Geometry check sheet. Reference: the model listing, model coordinates, mm. Coordinates: 2 decimals unless noted, no trailing zeros. Write each loop counter-clockwise with the first axis right and the second up, starting at its lowest first coordinate (ties: lowest second). Pieces come first, ordered by that corner, then holes. Notation, with made-up numbers: M 88.5,48.5 L 139.5,48.5 A23 ccw 139.5,56.5 Z; hole C 77.5,71.5 d8. An arc over 180 degrees is marked long. Answer as a JSON object with one key per item and string values. Group by question number.
Autodesk Inventor part; units mm, degrees
ref_plane "YZ Plane" through (0, 0, 0) normal (1, 0, 0) x (0, 1, 0)
ref_plane "XZ Plane" through (0, 0, 0) normal (0, 1, 0) x (-1, 0, 0)
ref_plane "XY Plane" through (0, 0, 0) normal (0, 0, 1) x (1, 0, 0)
sketch "Sketch1" plane through (0, 0, 0) normal (0, 0, 1) x (1, 0, 0)
  line L0 (0, 0) -> (101.6, 0)
  line L1 (101.6, 0) -> (101.6, 50.8)
  line L2 (0, 50.8) -> (0, 0)
  line L3 (50.8, 152.4) -> (0, 152.4)
  line L4 (0, 152.4) -> (0, 50.8)
  line L5 (50.8, 152.4) -> (101.6, 50.8)
  circle A0 centre (12.7, 12.7) radius 3.2512
  circle A1 centre (12.7, 38.1) radius 3.2512
  circle A2 centre (12.7, 63.5) radius 3.2512
  circle A3 centre (12.7, 88.9) radius 3.2512
  circle A4 centre (12.7, 114.3) radius 3.2512
  circle A5 centre (12.7, 139.7) radius 3.2512
  circle A6 centre (38.1, 12.7) radius 3.2512
  circle A7 centre (38.1, 38.1) radius 3.2512
  circle A8 centre (38.1, 63.5) radius 3.2512
  circle A9 centre (38.1, 88.9) radius 3.2512
  circle A10 centre (38.1, 114.3) radius 3.2512
  circle A11 centre (38.1, 139.7) radius 3.2512
  circle A12 centre (63.5, 12.7) radius 3.2512
  circle A13 centre (88.9, 12.7) radius 3.2512
  circle A14 centre (38.1, 38.1) radius 3.2512
  circle A15 centre (63.5, 38.1) radius 3.2512
  circle A16 centre (88.9, 38.1) radius 3.2512
  dimension "d6" = 101.6
  dimension "d7" = 50.8
  dimension "d8" = 50.8
  dimension "d9" = 101.6
  dimension "d10" = 50.8
  dimension "d11" = 101.6
  dimension "d12" = 50.8
  dimension "d13" = 6.5024
  dimension "d14" = 12.7
  dimension "d15" = 12.7
  dimension "d18" = 25.4
  dimension "d21" = 25.4
  dimension "d26" = 25.4
  dimension "d29" = 25.4
extrude "Extrusion1" add sketch "Sketch1" along normal blind 6.35
properties part number "6x4"
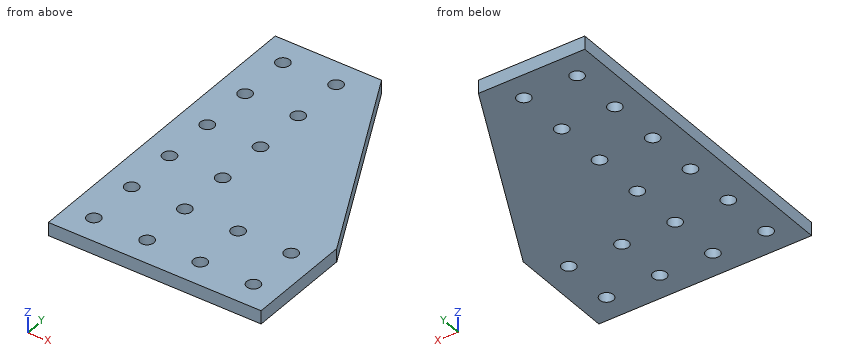
1) Material ranges on probe 1 along Y at (x, z) = (62, 4); probe 2 along Y at (x, z) = (78, 2.25); probe 3 along Y at (x, z) = (77, 1.75), recorded low to high. Write a range as [from, to].
2) Section check A-A (y = 12.7). Record the cut outline in (x, z), then the cut area to 3 significant figures.
3) Section check B-B (x = 63.5). Record the cut outline in (y, z), then the cut area to 3 significant figures.
4) Section check C-C (y = 63.5). Record the cut outline in (x, z), then the cut area to 3 significant figures.
5) Section check D-D (z = 2.25). State how many separate pieces and enclosed holes the cut face has, then the cut area to 3 significant figures.
Entries:
{
 "1": {"probe 1": "[0, 9.82], [15.58, 35.22], [40.98, 130]", "probe 2": "[0, 98]", "probe 3": "[0, 100]"},
 "2": {"outline": "M 0,0 L 9.45,0 L 9.45,6.35 L 0,6.35 Z; M 15.95,0 L 34.85,0 L 34.85,6.35 L 15.95,6.35 Z; M 41.35,0 L 60.25,0 L 60.25,6.35 L 41.35,6.35 Z; M 66.75,0 L 85.65,0 L 85.65,6.35 L 66.75,6.35 Z; M 92.15,0 L 101.6,0 L 101.6,6.35 L 92.15,6.35 Z", "area": "480 mm^2"},
 "3": {"outline": "M 0,0 L 9.45,0 L 9.45,6.35 L 0,6.35 Z; M 15.95,0 L 34.85,0 L 34.85,6.35 L 15.95,6.35 Z; M 41.35,0 L 127,0 L 127,6.35 L 41.35,6.35 Z", "area": "724 mm^2"},
 "4": {"outline": "M 0,0 L 9.45,0 L 9.45,6.35 L 0,6.35 Z; M 15.95,0 L 34.85,0 L 34.85,6.35 L 15.95,6.35 Z; M 41.35,0 L 95.25,0 L 95.25,6.35 L 41.35,6.35 Z", "area": "522 mm^2"},
 "5": {"separate pieces": "1", "enclosed holes": "16", "area": "12,400 mm^2"}
}
